from build123d import *

# Parameters (mm, degrees)
F0_W      = 18
F0_H      = 6
F1_DEPTH  = 3
F2_R      = 3
F2_R_2    = 2
F3_DEPTH  = 10
F4_R      = 1
F4_R_2    = 1.15
F5_DEPTH  = 20
F6_SIZE2  = 1.5
F6_SIZE   = 0.6
F7_W      = 11.6012076614
F7_H      = 11.8295210414
F8_DEPTH  = 7
F9_R      = 2.9999
F10_R     = 2.55
F10_R_2   = 1
F11_DEPTH = 1.5


# Not quite as in the source:
# - a fillet or chamfer is up to 0.001 mm smaller than in the source, because OpenCascade refuses the exact size


with BuildPart() as f1:
    # F0 (on Top) → F1 (new body)
    with BuildSketch(Plane.XY):
        with Locations((1.8924829921, 0)):
            Rectangle(F0_W, F0_H)
    extrude(amount=F1_DEPTH)

    # F2 (on face) → F3 (join)
    with BuildSketch(Plane.XY.offset(3)):
        with Locations((7.8924829921, 0)):
            Circle(F2_R)
        with Locations((-4.1075170079, 0)):
            Circle(F2_R_2)
    extrude(amount=F3_DEPTH)

    # F4 (on face) → F5 (cut)
    with BuildSketch(Plane.XY.offset(13)):
        with Locations((-4.1075170079, 0)):
            Circle(F4_R)
        with Locations((7.8924829921, 0)):
            Circle(F4_R_2)
    extrude(amount=-F5_DEPTH, mode=Mode.SUBTRACT)

    # F6
    f6_edges = [f1.edges().sort_by_distance(p)[0] for p in [
        (-6.107517, 0, 13),
    ]]
    f6_side = f1.faces().sort_by_distance((-6.050948, 0, 13))[0]
    chamfer(f6_edges, length=F6_SIZE, length2=F6_SIZE2, reference=f6_side)

    # F7 (on face) → F8 (cut)
    with BuildSketch(Plane.XY.offset(13)):
        with Locations((7.5882198871, -0.5373002496)):
            Rectangle(F7_W, F7_H)
    extrude(amount=-F8_DEPTH, mode=Mode.SUBTRACT)

    # F9 (radius 3 in the source; OpenCascade refuses exactly that, so slightly less here)
    f9_edges = [f1.edges().sort_by_distance(p)[0] for p in [
        (10.892483, -3, 1.5),
        (10.892483, 3, 1.5),
        (-7.107517, 3, 1.5),
        (-7.107517, -3, 1.5),
    ]]
    fillet(f9_edges, radius=F9_R)

    # F10 (on face) → F11 (cut)
    with BuildSketch(Plane(origin=(0, 0, 0), x_dir=(1, 0, 0), z_dir=(0, 0, -1))):
        with Locations((-4.1075170079, 0)):
            Circle(F10_R)
        with Locations((-4.1075170079, 0)):
            Circle(F10_R_2, mode=Mode.SUBTRACT)
    extrude(amount=-F11_DEPTH, mode=Mode.SUBTRACT)


solid = f1.part
Build history of the part. All positions in model axes, mm. A direction names the side the tool comes from. Round coordinates to 2 decimals unless told otherwise and drop trailing zeros. Loops run counter-clockwise (first coordinate to the right, second up) from the corner with the lowest first, then second, coordinate; pieces in that order, holes last. Notation, with made-up numbers: (39, 30.25) -> (53, 30.25) arc R17 ccw to (53, 51.25) -> close; hole circle Ø10 at (28, 38). An arc over 180 degrees is marked (long way). One line per item, written item: value. Start each with the question number.
Q1. 3-axis set-ups, long thin cutter, end or side, ignore diameter. For faces 1 (the face through (-3.184, -0.383, 7.33)), 2 (the face through (7.9, -1.3, 6)), 3 (the face through (-3.6, 1.1, 1.5)), 4 (the face through (2, 3, 1)), 5 (the face through (-2.26, -0.77, 7.19)): which of +Z, -Z, +X, -X, +Y, -Y reach the whole face in a straight line?
Q2. Cut at D-D on z = 8.5. List the corners of the cut face in (x, y), plus the area to 3 significant figures.
Q3. Drop flat-ended pins along their axis: pin 1 Ø3 at (x, y) = (6.5, 0) entering from +Z; pin 2 Ø1.6 at (x, y) = (-4.11, 0) entering from -Z; pin 3 Ø2 at (y, z) = (-1, 4) entering from +X; pin 4 Ø1.8 at (x, y) = (-1, -1) entering from +Z. Give the stop position or say it passes through.
Q4. Two-plate mould, pull along X, no slides. Class faces 6 (the face through (-1.675, -0.766, 0.74)), 7 (the face through (2, -3, 1)), 8 (the face through (9.99, -2.145, 1.521)): released by +X, released by -X, zero draft, split by the parting line, or undercut.
Q5. Probe line 1 along X through (y, z) = (-0.75, 5.25); line 2 along Z through (x, y) = (7, 2.5); line 3 along Z through (x, y) = (4.5, -2). List the from-to ranges inside material, lowest first.
Q6. Cut at C-C on x = 5.5. List the corners of the cut face in (y, z), plus the area to 3 significant figures.
Q7. Cut at A-A on z = 2.75. Count the separate pieces of the cut face and the enclosed holes in it, plus the area to 3 significant figures.
Computed:
1. face 1: +Z, -Z
1. face 2: +Z, +X, +Y, -Y
1. face 3: -Z
1. face 4: +Z, -Z, +X, -X, +Y
1. face 5: +Z
2. outline: circle Ø4 at (-4.11, 0); hole circle Ø2 at (-4.11, 0)
2. area: 9.42 mm²
3. pin 1: z = 6
3. pin 2: through
3. pin 3: x = 10.89
3. pin 4: z = 3
4. face 6: undercut
4. face 7: zero draft
4. face 8: released by +X
5. line 1: -5.96 to -4.77, -3.45 to -2.25, 4.99 to 7.02, 8.76 to 10.8
5. line 2: 0 to 6
5. line 3: 0 to 3
6. outline: (-3, 0) -> (3, 0) -> (3, 3) -> (1.81, 3) -> (1.81, 6) -> (-1.81, 6) -> (-1.81, 3) -> (-3, 3) -> close
6. area: 28.9 mm²
7. separate pieces: 1
7. enclosed holes: 2
7. area: 93.0 mm²
